from build123d import *

# Parameters (mm, degrees)
BOSS_EXTRUDE1_DEPTH     = 27.94
SKETCH2_R               = 3.5306
SKETCH2_R_2             = 1.4986
SKETCH2_R_3             = 2.032
MOTOR_MOUNT_HOLES_DEPTH = 52.022252766
SKETCH3_R               = 1.651
PLATE_MOUNT_HOLES_DEPTH = 52.022252766
FILLET1_R               = 0.635
FILLET2_R               = 0.889
FILLET3_R               = 0.635


with BuildPart() as part:
    # Sketch1 → Boss-Extrude1 (new body)
    with BuildSketch(Plane(origin=(0, 0, 0), x_dir=(0, 0, -1), z_dir=(1, 0, 0))):
        Polygon((0, 0), (0, -30.1244), (-30.2514, -30.1244), (-30.2514, -27.0256), (-3.1496, -27.0256), (-3.1496, 0), align=None)
    extrude(amount=BOSS_EXTRUDE1_DEPTH)

    # Sketch2 → Motor_Mount_holes (cut, through all)
    with BuildSketch(Plane.XY):
        with Locations(Location((13.97, -12.1666, 0), (0, 0, 90))):
            Circle(SKETCH2_R)
        with Locations(Location((13.97, -4.5212, 0), (0, 0, 90))):
            Circle(SKETCH2_R_2)
        with Locations(Location((5.2705, -12.1666, 0), (0, 0, 90))):
            Circle(SKETCH2_R_3)
        with Locations(Location((22.6695, -12.1666, 0), (0, 0, 180))):
            Circle(SKETCH2_R_3)
        with Locations(Location((13.97, -19.812, 0), (0, 0, 180))):
            Circle(SKETCH2_R_2)
    extrude(amount=MOTOR_MOUNT_HOLES_DEPTH, mode=Mode.SUBTRACT)

    # Sketch3 → Plate_Mount_Holes (cut, through all)
    with BuildSketch(Plane(origin=(0, -30.1244, 0), x_dir=(1, 0, 0), z_dir=(0, 1, 0))):
        with Locations(Location((3.937, -7.747, 0), (0, 0, 90))):
            Circle(SKETCH3_R)
        with Locations(Location((23.876, -7.747, 0), (0, 0, 90))):
            Circle(SKETCH3_R)
        with Locations(Location((3.937, -21.2598, 0), (0, 0, 90))):
            Circle(SKETCH3_R)
        with Locations(Location((23.876, -21.2598, 0), (0, 0, 90))):
            Circle(SKETCH3_R)
    extrude(amount=PLATE_MOUNT_HOLES_DEPTH, mode=Mode.SUBTRACT)

    # Fillet1
    fillet1_edges = [part.edges().sort_by_distance(p)[0] for p in [
        (13.97, -27.0256, 3.1496),
    ]]
    fillet(fillet1_edges, radius=FILLET1_R)

    # Fillet2
    fillet2_edges = [part.edges().sort_by_distance(p)[0] for p in [
        (13.97, -30.1244, 0),
    ]]
    fillet(fillet2_edges, radius=FILLET2_R)

    # Fillet3
    fillet3_edges = [part.edges().sort_by_distance(p)[0] for p in [
        (13.97, 0, 0),
        (13.97, -30.1244, 30.2514),
        (13.97, -27.0256, 30.2514),
        (13.97, 0, 3.1496),
    ]]
    fillet(fillet3_edges, radius=FILLET3_R)


solid = part.part
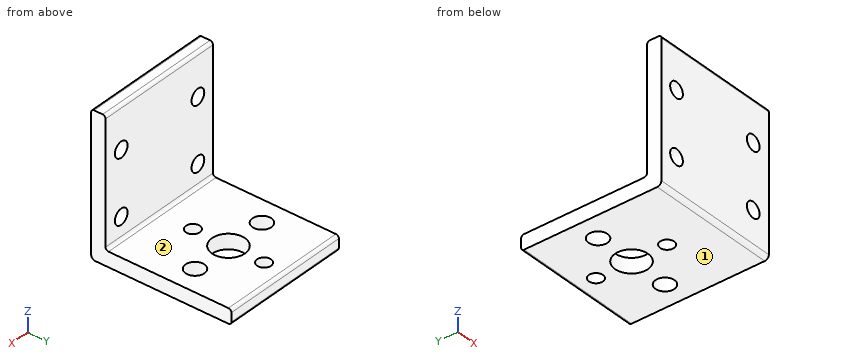
Geometry: final body of the model. Coordinates: model frame, mm. Face numbers are marked on the shaded views. A direction names the side the tool comes from. Coordinates: 2 decimals unless noted, no trailing zeros. Order: outer loops, then holes, each group sorted by start corner. A loop starts at its lowest first (then second) coordinate and runs counter-clockwise, first axis right, second up. Notation, with made-up numbers: M 42.25,-39.75 L 88.25,-39.75 A26 cw 88.25,-13.75 Z; hole C -20,48 d1. An arc over 180 degrees is marked long. One line per question, with ' | ' between items. Start each with the question number.
Item 1: Cut plane B-B, the plane z = 22. Return the cut outline in (x, y), then the cut area to 3 significant figures.
Item 2: Ray query, probe 1 along Y at (x, z) = (13.97, 1.6); probe 2 along Z at (x, y) = (4.25, -8.5); probe 3 along Y at (x, z) = (8, 23). Return the intervals inside material, ascending. Write a range as [from, to].
Item 3: Cut plane C-C, the plane x = 8.75. Return the cut outline in (y, z) (3 decimals), then the cut area to 3 significant figures.
Item 4: Cut plane D-D, the plane z = 28. Return the cut outline in (x, y), then the cut area to 3 significant figures.
Item 5: Cut plane A-A, the plane x = 13.97. Return the cut outline in (y, z) (3 decimals), then the cut area to 3 significant figures.
Item 6: Set-up query: the marked faces 1 and 2. Return all of +Z, -Z, +X, -X, +Y, -Y with unobstructed straight access to the full face (end or side cutting, diameter ignored); none if empty.
Item 7: Pin query (flat end, axial travel): pin 1 Ø7.5 at (x, y) = (18, -8) entering from +Z; pin 2 Ø8 at (x, z) = (4.5, 25) entering from +Y. Return the tip coordinate at first contact, or that it passes through.
A:
1) outline: M 0,-30.12 L 2.46,-30.12 L 2.46,-27.03 L 0,-27.03 Z; M 5.41,-30.12 L 22.4,-30.12 L 22.4,-27.03 L 5.41,-27.03 Z; M 25.35,-30.12 L 27.94,-30.12 L 27.94,-27.03 L 25.35,-27.03 Z | area: 68.3 mm2
2) probe 1: y = [-30.12, -21.31], [-18.31, -15.7], [-8.64, -6.02], [-3.02, 0] | probe 2: z = [0, 3.15] | probe 3: y = [-30.12, -27.03]
3) outline: M -30.124,0.889 A0.889 ccw -29.235,0 L -0.635,0 A0.635 ccw 0,0.635 L 0,2.515 A0.635 ccw -0.635,3.15 L -26.391,3.15 A0.635 cw -27.026,3.785 L -27.026,29.616 A0.635 ccw -27.661,30.251 L -29.489,30.251 A0.635 ccw -30.124,29.616 Z | area: 178 mm2
4) outline: M 0,-30.12 L 27.94,-30.12 L 27.94,-27.03 L 0,-27.03 Z | area: 86.6 mm2
5) outline: M -30.124,0.889 A0.889 ccw -29.235,0 L -21.311,0 L -21.311,3.15 L -26.391,3.15 A0.635 cw -27.026,3.785 L -27.026,29.616 A0.635 ccw -27.661,30.251 L -29.489,30.251 A0.635 ccw -30.124,29.616 Z; M -18.313,0 L -15.697,0 L -15.697,3.15 L -18.313,3.15 Z; M -8.636,0 L -6.02,0 L -6.02,3.15 L -8.636,3.15 Z; M -3.023,0 L -0.635,0 A0.635 ccw 0,0.635 L 0,2.515 A0.635 ccw -0.635,3.15 L -3.023,3.15 Z | area: 137 mm2
6) face 1: -Z, +X, -X, +Y, -Y | face 2: +Z, +X, -X, +Y
7) pin 1: stops at z = 3.15 | pin 2: stops at y = -27.03
